```python
from build123d import *

# Parameters (mm, degrees)
CROQUIS1_R              = 110
SALIENTE_EXTRUIR1_DEPTH = 10
CORTAR_EXTRUIR2_DEPTH   = 156.884572681
CROQUIS5_R              = 4
CORTAR_EXTRUIR3_DEPTH   = 156.884572681


with BuildPart() as part:
    # Croquis1 → Saliente-Extruir1 (new body)
    with BuildSketch(Plane(origin=(0, 0, 0), x_dir=(1, 0, 0), z_dir=(0, 1, 0))):
        with Locations(Location((0, 0, 0), (0, 0, 270))):
            Circle(CROQUIS1_R)
    extrude(amount=SALIENTE_EXTRUIR1_DEPTH)

    # Croquis3 → Cortar-Extruir2 (cut, through all)
    with BuildSketch(Plane(origin=(0, 10, 0), x_dir=(1, 0, 0), z_dir=(0, 1, 0))):
        with BuildLine():
            Line((-19.635517807, 1.200433086), (-16.643149179, 1.41427881))
            ThreePointArc((-16.643149179, 1.41427881), (-13.867597162, -0.991029758), (-16.27290573, -3.766581775))
            Line((-16.27290573, -3.766581775), (-19.265274358, -3.980427499))
            ThreePointArc((-19.265274358, -3.980427499), (-22.040826375, -1.575118931), (-19.635517807, 1.200433086))
        make_face()
        with BuildLine():
            Line((16.244753287, 3.783863744), (19.237121915, 4.028597389))
            ThreePointArc((19.237121915, 4.028597389), (22.058108344, 1.634159295), (19.66367025, -1.186827134))
            Line((19.66367025, -1.186827134), (16.671301622, -1.431560779))
            ThreePointArc((16.671301622, -1.431560779), (13.850315193, 0.962877315), (16.244753287, 3.783863744))
        make_face()
    extrude(amount=-CORTAR_EXTRUIR2_DEPTH, mode=Mode.SUBTRACT)

    # Croquis5 → Cortar-Extruir3 (cut, through all)
    with BuildSketch(Plane(origin=(0, 10, 0), x_dir=(1, 0, 0), z_dir=(0, 1, 0))):
        with Locations(Location((-85.209654188, -52.338464184, 0), (0, 0, 270))):
            Circle(CROQUIS5_R)
        with Locations(Location((-97.26120724, 23.243441358, 0), (0, 0, 270))):
            Circle(CROQUIS5_R)
        with Locations(Location((-52.338464184, 85.209654188, 0), (0, 0, 270))):
            Circle(CROQUIS5_R)
        with Locations(Location((23.243441358, 97.26120724, 0), (0, 0, 270))):
            Circle(CROQUIS5_R)
        with Locations(Location((85.209654188, 52.338464184, 0), (0, 0, 270))):
            Circle(CROQUIS5_R)
        with Locations(Location((97.26120724, -23.243441358, 0), (0, 0, 270))):
            Circle(CROQUIS5_R)
        with Locations(Location((52.338464184, -85.209654188, 0), (0, 0, 270))):
            Circle(CROQUIS5_R)
        with Locations(Location((-23.243441358, -97.26120724, 0), (0, 0, 270))):
            Circle(CROQUIS5_R)
    extrude(amount=-CORTAR_EXTRUIR3_DEPTH, mode=Mode.SUBTRACT)


solid = part.part
```
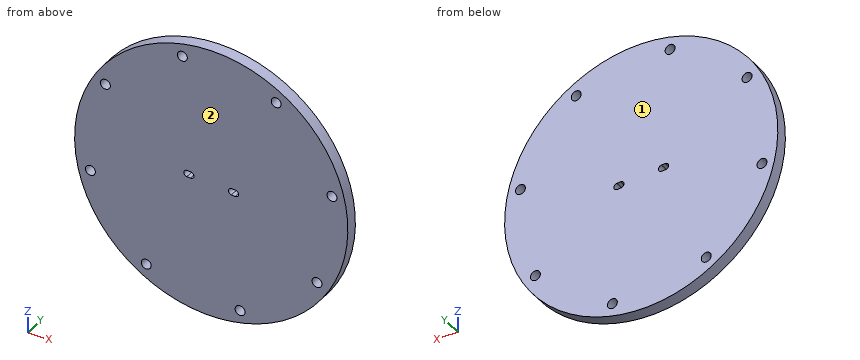
Design review of the part built by this model. Coordinates are the model's own, in mm. Face numbers are marked on the shaded views. Give positions to 0.01 mm unless a question says otherwise; leave off trailing zeros. Write each loop counter-clockwise with the first axis right and the second up, starting at its lowest first coordinate (ties: lowest second). Pieces come first, ordered by that corner, then holes.
(1) Add section A-A (y = 4.25). Give the number of separate pieces and of enclosed holes in the cut face, and give its area (3 significant figures).
Checked values:
separate pieces: 1
enclosed holes: 10
area: 37,500 mm2
(2) Wall thickness on line 1 along Z through (x, y) = (2, 7.25); line 2 along Z through (x, y) = (53, 1); line 3 along Z through (x, y) = (-50.5, 8.75): over which ranges is each line inside the solid? List them lowest first.
Checked values:
line 1: z = -109.98 to 109.98
line 2: z = -96.39 to 81.26, 89.15 to 96.39
line 3: z = -97.72 to -88.76, -81.66 to 97.72
(3) Add section C-C (x = 63). Give the boundary of the cut face in (y, z).
Checked values:
outline: (0, -90.17) - (10, -90.17) - (10, 90.17) - (0, 90.17) - close
(4) Add section B-B (z = 32.5). Give the boundary of the cut face in (x, y).
Checked values:
outline: (-105.09, 0) - (105.09, 0) - (105.09, 10) - (-105.09, 10) - close
(5) Mouldability with a two-part tool opening along Y and no side actions: class the marked faces 1 and 2 as +Y half, -Y half, draft (parallel to the pull), parting line (faces both ways), or undercut.
Checked values:
face 1: +Y half
face 2: -Y half
(6) Clearance check with flat-ended pins moving along their axes: pin 1 Ø4 at (y, z) = (8.5, 55.5) entering from +X; pin 2 Ø6 at (y, z) = (7.5, -33) entering from -X; pin 3 Ø3 at (y, z) = (8, -13) entering from +X. State where each tip first meets the part, or that it passes through.
Checked values:
pin 1: stops at x = 96.11
pin 2: stops at x = -105.83
pin 3: stops at x = 109.4
